Design review of the part built by this model. Coordinates are the model's own, in mm. Face numbers are marked on the shaded views. A direction names the side the tool comes from. Coordinates: 2 decimals unless noted, no trailing zeros. Loops run counter-clockwise (first coordinate to the right, second up) from the corner with the lowest first, then second, coordinate; pieces in that order, holes last. Notation, with made-up numbers: (38, 35) -> (71, 35) arc R31 ccw to (71, 74) -> close; hole circle Ø9 at (-20.5, 60). An arc over 180 degrees is marked (long way). One line per item, written item: value. Start each with the question number.
1. Add section C-C on z = 22.5. Write out the cut boundary in (x, y).
2. Add section A-A on z = 7.5. Write out the cut boundary in (x, y), plus the area to 3 significant figures.
3. Machinability: for the marked faces 5, 6, 7 and 8, which of the approach directions +Z, -Z, +X, -X, +Y, -Y give a long, thin tool a straight path to every point of the face, cutting with its end or side? Answer none if there is none.
4. Insertion check: pin 1 (12 mm diameter, centred on y = -15.5, z = 5.5, fed in from -X); pin 2 (17.5 mm diameter, centred on x = 0.5, y = -21.5, fed in from +Z); pin 3 (18 mm diameter, centred on x = 0, y = 0, fed in from +Z); pin 4 (6 mm diameter, centred on x = -0.5, z = 6, fed in from -Y). Each pin has a flat end and moves straight along its axis. Give the tip position at first contact, or say it passes through.
5. Draft analysis for pull direction X (two halves, no side actions). For the marked faces 1, 2, 3 and 4, state which applies: pulls with the +X half, pulls with the -X half, needs draft (parallel to the pull), parting line crosses it, or undercut.
6. For probe 1 along Z at (x, y) = (-25, -78.6); probe 2 along X at (y, z) = (-26, 14.5); probe 3 along X at (y, z) = (2, 2), list the stretches that pass through material, from the lowest coordinate up.
7. Add section B-B on x = -25. Write out the cut boundary in (y, z).
8. Add section D-D on y = -23.5. Write out the cut boundary in (x, z), plus the area to 3 significant figures.
```python
from build123d import *

# Parameters (mm, degrees)
BOSS_EXTRUDE1_DEPTH = 15
BOSS_EXTRUDE3_START = 1
BOSS_EXTRUDE3_DEPTH = 1
SKETCH7_W           = 15
SKETCH7_H           = 9
BOSS_EXTRUDE4_DEPTH = 15
FILLET1_R           = 1
CHAMFER1_SIZE       = 2.5
CHAMFER2_SIZE       = 1


with BuildPart() as part:
    # Sketch1 → Boss-Extrude1 (new body)
    with BuildSketch(Plane.XY):
        with BuildLine():
            Line((-8.5, -71), (17.5, -30))
            Line((17.5, -30), (17.5, 0))
            ThreePointArc((17.5, 0), (13.795379661, 10.767427734), (4.25, 16.976086121))
            Line((4.25, 16.976086121), (4.25, 10.145811944))
            ThreePointArc((4.25, 10.145811944), (0, -11), (-4.25, 10.145811944))
            Line((-4.25, 10.145811944), (-4.25, 16.976086121))
            ThreePointArc((-4.25, 16.976086121), (-13.795379661, 10.767427734), (-17.5, 0))
            Line((-17.5, 0), (-17.5, -71))
            Line((-17.5, -71), (-32.5, -71))
            Line((-32.5, -71), (-32.5, -80))
            Line((-32.5, -80), (-8.5, -80))
            Line((-8.5, -80), (-8.5, -71))
        make_face()
        Polygon((8.5, -17.5), (8.5, -30), (-8.5, -56.807692308), (-8.5, -17.5), align=None, mode=Mode.SUBTRACT)
    extrude(amount=BOSS_EXTRUDE1_DEPTH)

    # Sketch6 → Boss-Extrude3 (add)
    with BuildSketch(Plane(origin=(0, 0, 15), x_dir=(-1, 0, 0), z_dir=(0, 0, -1)).offset(BOSS_EXTRUDE3_START)):
        with BuildLine():
            Line((-4.25, 9.051933495), (-4.25, 10.145811944))
            ThreePointArc((-4.25, 10.145811944), (-6.093028803, -9.158329542), (11, 0))
            ThreePointArc((11, 0), (9.158329542, 6.093028803), (4.25, 10.145811944))
            Line((4.25, 10.145811944), (4.25, 9.051933495))
            ThreePointArc((4.25, 9.051933495), (8.440971508, 5.361902647), (10, 0))
            ThreePointArc((10, 0), (-5.361902647, -8.440971508), (-4.25, 9.051933495))
        make_face()
    extrude(amount=-BOSS_EXTRUDE3_DEPTH)

    # Sketch7 → Boss-Extrude4 (add)
    with BuildSketch(Plane.XY.offset(15)):
        with Locations((-16, -75.5)):
            Rectangle(SKETCH7_W, SKETCH7_H)
    extrude(amount=BOSS_EXTRUDE4_DEPTH)

    # Sketch11 → Cut-Revolve4 (revolve, cut)
    with BuildSketch(Plane.ZY.offset(25)):
        Polygon((7.5, -71), (7.5, -80), (9.7, -80), (9.7, -74), (12.307860213, -71), align=None)
    revolve(axis=Axis((-25, -71, 7.5), (0, -1, 0)), mode=Mode.SUBTRACT)

    # Sketch10 → Cut-Revolve3 (revolve, cut)
    with BuildSketch(Plane.XY.offset(22.5), mode=Mode.PRIVATE) as cut_revolve3_sk:
        Polygon((-16, -71), (-11.192139787, -71), (-13.8, -74), (-13.8, -80), (-16, -80), align=None)
    revolve(cut_revolve3_sk.sketch.rotate(Axis((-16, -80, 22.5), (0, 1, 0)), 90), axis=Axis((-16, -80, 22.5), (0, 1, 0)), mode=Mode.SUBTRACT)

    # Fillet1
    fillet1_edges = [part.edges().sort_by_distance(p)[0] for p in [
        (0, -11, 0),
    ]]
    fillet(fillet1_edges, radius=FILLET1_R)

    # Chamfer1
    chamfer1_edges = [part.edges().sort_by_distance(p)[0] for p in [
        (-32.5, -75.5, 0),
        (-8.5, -17.5, 7.5),
        (8.5, -17.5, 7.5),
        (-32.5, -75.5, 15),
        (-23.5, -75.5, 30),
        (-8.5, -75.5, 30),
    ]]
    chamfer(chamfer1_edges, length=CHAMFER1_SIZE)

    # Chamfer2
    chamfer2_edges = [part.edges().sort_by_distance(p)[0] for p in [
        (0, -10, 14),
    ]]
    chamfer(chamfer2_edges, length=CHAMFER2_SIZE - 0.0001)  # a hair under: the kernel refuses the full size


solid = part.part
```
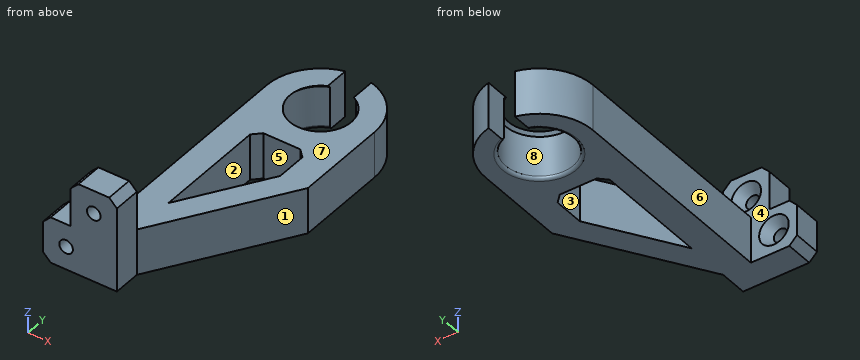
Worked answers:
1. outline: (-23.5, -80) -> (-18.2, -80) -> (-18.2, -74) -> (-20.81, -71) -> (-23.5, -71) -> close; (-13.8, -80) -> (-8.5, -80) -> (-8.5, -71) -> (-11.19, -71) -> (-13.8, -74) -> close
2. outline: (-32.5, -80) -> (-27.2, -80) -> (-27.2, -74) -> (-29.81, -71) -> (-32.5, -71) -> close; (-22.8, -80) -> (-8.5, -80) -> (-8.5, -71) -> (17.5, -30) -> (17.5, 0) arc R17.5 ccw to (4.25, 16.98) -> (4.25, 10.15) arc R11 cw (long way) to (-4.25, 10.15) -> (-4.25, 16.98) arc R17.5 ccw to (-17.5, 0) -> (-17.5, -71) -> (-20.19, -71) -> (-22.8, -74) -> close; hole (-8.5, -56.81) -> (8.5, -30) -> (8.5, -20) -> (6, -17.5) -> (-6, -17.5) -> (-8.5, -20) -> close
2. area: 1,730 mm²
3. face 5: +Z, -Z
3. face 6: +Z, -Z, -X, +Y
3. face 7: +Z, +X, -X, +Y
3. face 8: -Z
4. pin 1: stops at x = -17.5
4. pin 2: stops at z = 15
4. pin 3: passes through
4. pin 4: stops at y = -63.12
5. face 1: pulls with the +X half
5. face 2: undercut
5. face 3: undercut
5. face 4: needs draft
6. probe 1: z = 0 to 5.3, 9.7 to 15
6. probe 2: x = -17.5 to -8.5, 8.5 to 17.5
6. probe 3: x = -17.39 to -10.82, 10.82 to 17.39
7. outline: (-80, 0) -> (-71, 0) -> (-71, 2.69) -> (-74, 5.3) -> (-80, 5.3) -> close; (-80, 9.7) -> (-74, 9.7) -> (-71, 12.31) -> (-71, 15) -> (-80, 15) -> close
8. outline: (-17.5, 0) -> (-8.5, 0) -> (-8.5, 15) -> (-17.5, 15) -> close; (8.5, 0) -> (17.5, 0) -> (17.5, 15) -> (8.5, 15) -> close
8. area: 270 mm²
